```python
from build123d import *

# Parameters (mm, degrees)
SKETCH1_W           = 99
SKETCH1_H           = 126
BOSS_EXTRUDE1_DEPTH = 3
FILLET1_R           = 5
SKETCH5_R           = 18.5
SKETCH5_R_2         = 2.5
CUT_EXTRUDE4_DEPTH  = 81.176368089
SKETCH2_R           = 1.75
CUT_EXTRUDE1_DEPTH  = 81.176368089
CHAMFER1_SIZE       = 0.5
FILLET3_R           = 2
CUT_EXTRUDE3_DEPTH  = 81.176368089
SKETCH3_W           = 13.330399243
SKETCH3_H           = 8
CUT_EXTRUDE2_DEPTH  = 81.176368089
FILLET2_R           = 2.5


with BuildPart() as part:
    # Sketch1 → Boss-Extrude1 (new body)
    with BuildSketch(Plane(origin=(0, 0, 0), x_dir=(1, 0, 0), z_dir=(0, 1, 0))):
        Rectangle(SKETCH1_W, SKETCH1_H)
    extrude(amount=BOSS_EXTRUDE1_DEPTH)

    # Fillet1
    fillet1_edges = [part.edges().sort_by_distance(p)[0] for p in [
        (49.5, 1.5, 63),
        (-49.5, 1.5, 63),
        (-49.5, 1.5, -63),
        (49.5, 1.5, -63),
    ]]
    fillet(fillet1_edges, radius=FILLET1_R)

    # Sketch5 → Cut-Extrude4 (cut, through all)
    with BuildSketch(Plane(origin=(0, 3, 0), x_dir=(1, 0, 0), z_dir=(0, 1, 0))):
        with Locations(Location((0, 28, 0), (0, 0, 270))):
            Circle(SKETCH5_R)
        with Locations(Location((16, 44, 0), (0, 0, 270))):
            Circle(SKETCH5_R_2)
        with Locations(Location((16, 12, 0), (0, 0, 90))):
            Circle(SKETCH5_R_2)
        with Locations(Location((-16, 12, 0), (0, 0, 270))):
            Circle(SKETCH5_R_2)
        with Locations(Location((-16, 44, 0), (0, 0, 90))):
            Circle(SKETCH5_R_2)
    extrude(amount=-CUT_EXTRUDE4_DEPTH, mode=Mode.SUBTRACT)

    # Sketch2 → Cut-Extrude1 (cut, through all)
    with BuildSketch(Plane(origin=(0, 3, 0), x_dir=(1, 0, 0), z_dir=(0, 1, 0))):
        with Locations(Location((-43, 56.5, 0), (0, 0, 270))):
            Circle(SKETCH2_R)
        with Locations(Location((43, 56.5, 0), (0, 0, 90))):
            Circle(SKETCH2_R)
        with Locations(Location((43, -56.5, 0), (0, 0, 270))):
            Circle(SKETCH2_R)
        with Locations(Location((-43, -56.5, 0), (0, 0, 90))):
            Circle(SKETCH2_R)
    extrude(amount=-CUT_EXTRUDE1_DEPTH, mode=Mode.SUBTRACT)

    # Chamfer1
    chamfer1_edges = [part.edges().sort_by_distance(p)[0] for p in [
        (-16, 3, -41.5),
        (-16, 3, -14.5),
        (16, 3, -9.5),
        (16, 3, -46.5),
    ]]
    chamfer(chamfer1_edges, length=CHAMFER1_SIZE)

    # Fillet3
    # the kernel refuses this fillet: 2 mm, written as the material it takes off along each edge
    with BuildSketch(Plane(origin=(0, 3, -28), x_dir=(0, 0, 1), z_dir=(-1, 0, 0))) as fillet3_piece_1:
        with BuildLine():
            CenterArc((18.5 + FILLET3_R, -FILLET3_R), FILLET3_R, 90, 90)
            Line((18.5, -FILLET3_R), (18.5, 0))
            Line((18.5, 0), (18.5 + FILLET3_R, 0))
        make_face()
    revolve(axis=Axis((0, 3, -28), (0, 1, 0)), mode=Mode.SUBTRACT)

    # Sketch4 → Cut-Extrude3 (cut, through all)
    with BuildSketch(Plane(origin=(0, 3, 0), x_dir=(1, 0, 0), z_dir=(0, 1, 0))):
        with BuildLine():
            Line((-39.5, -48.833333333), (-5, -48.833333333))
            ThreePointArc((-5, -48.833333333), (-2.5, -51.333333333), (-5, -53.833333333))
            Line((-5, -53.833333333), (-39.5, -53.833333333))
            ThreePointArc((-39.5, -53.833333333), (-42, -51.333333333), (-39.5, -48.833333333))
        make_face()
        with BuildLine():
            Line((-39.5, -39.5), (-5, -39.5))
            ThreePointArc((-5, -39.5), (-2.5, -42), (-5, -44.5))
            Line((-5, -44.5), (-39.5, -44.5))
            ThreePointArc((-39.5, -44.5), (-42, -42), (-39.5, -39.5))
        make_face()
        with BuildLine():
            Line((-39.5, -30.166666667), (-5, -30.166666667))
            ThreePointArc((-5, -30.166666667), (-2.5, -32.666666667), (-5, -35.166666667))
            Line((-5, -35.166666667), (-39.5, -35.166666667))
            ThreePointArc((-39.5, -35.166666667), (-42, -32.666666667), (-39.5, -30.166666667))
        make_face()
        with BuildLine():
            Line((-39.5, -20.833333333), (-5, -20.833333333))
            ThreePointArc((-5, -20.833333333), (-2.5, -23.333333333), (-5, -25.833333333))
            Line((-5, -25.833333333), (-39.5, -25.833333333))
            ThreePointArc((-39.5, -25.833333333), (-42, -23.333333333), (-39.5, -20.833333333))
        make_face()
        with BuildLine():
            Line((-39.5, -11.5), (-5, -11.5))
            ThreePointArc((-5, -11.5), (-2.5, -14), (-5, -16.5))
            Line((-5, -16.5), (-39.5, -16.5))
            ThreePointArc((-39.5, -16.5), (-42, -14), (-39.5, -11.5))
        make_face()
        with BuildLine():
            Line((-39.5, -2.166666667), (-5, -2.166666667))
            ThreePointArc((-5, -2.166666667), (-2.5, -4.666666667), (-5, -7.166666667))
            Line((-5, -7.166666667), (-39.5, -7.166666667))
            ThreePointArc((-39.5, -7.166666667), (-42, -4.666666667), (-39.5, -2.166666667))
        make_face()
        with BuildLine():
            Line((-39.5, 7.166666667), (-14.553540997, 7.166666667))
            ThreePointArc((-14.553540997, 7.166666667), (-12.053540997, 4.666666667), (-14.553540997, 2.166666667))
            Line((-14.553540997, 2.166666667), (-39.5, 2.166666667))
            ThreePointArc((-39.5, 2.166666667), (-42, 4.666666667), (-39.5, 7.166666667))
        make_face()
        with BuildLine():
            Line((-39.5, 16.5), (-23.669600757, 16.5))
            ThreePointArc((-23.669600757, 16.5), (-21.169600757, 14), (-23.669600757, 11.5))
            Line((-23.669600757, 11.5), (-39.5, 11.5))
            ThreePointArc((-39.5, 11.5), (-42, 14), (-39.5, 16.5))
        make_face()
        with BuildLine():
            Line((-39.5, 25.833333333), (-27.101147987, 25.833333333))
            ThreePointArc((-27.101147987, 25.833333333), (-24.601147987, 23.333333333), (-27.101147987, 20.833333333))
            Line((-27.101147987, 20.833333333), (-39.5, 20.833333333))
            ThreePointArc((-39.5, 20.833333333), (-42, 23.333333333), (-39.5, 25.833333333))
        make_face()
        with BuildLine():
            Line((-39.5, 35.166666667), (-27.101147987, 35.166666667))
            ThreePointArc((-27.101147987, 35.166666667), (-24.601147987, 32.666666667), (-27.101147987, 30.166666667))
            Line((-27.101147987, 30.166666667), (-39.5, 30.166666667))
            ThreePointArc((-39.5, 30.166666667), (-42, 32.666666667), (-39.5, 35.166666667))
        make_face()
        with BuildLine():
            Line((39.5, 44.5), (23.669600757, 44.5))
            ThreePointArc((23.669600757, 44.5), (21.169600757, 42), (23.669600757, 39.5))
            Line((23.669600757, 39.5), (39.5, 39.5))
            ThreePointArc((39.5, 39.5), (42, 42), (39.5, 44.5))
        make_face()
        with BuildLine():
            Line((-39.5, 44.5), (-23.669600757, 44.5))
            ThreePointArc((-23.669600757, 44.5), (-21.169600757, 42), (-23.669600757, 39.5))
            Line((-23.669600757, 39.5), (-39.5, 39.5))
            ThreePointArc((-39.5, 39.5), (-42, 42), (-39.5, 44.5))
        make_face()
        with BuildLine():
            Line((39.5, 35.166666667), (27.101147987, 35.166666667))
            ThreePointArc((27.101147987, 35.166666667), (24.601147987, 32.666666667), (27.101147987, 30.166666667))
            Line((27.101147987, 30.166666667), (39.5, 30.166666667))
            ThreePointArc((39.5, 30.166666667), (42, 32.666666667), (39.5, 35.166666667))
        make_face()
        with BuildLine():
            Line((39.5, 25.833333333), (27.101147987, 25.833333333))
            ThreePointArc((27.101147987, 25.833333333), (24.601147987, 23.333333333), (27.101147987, 20.833333333))
            Line((27.101147987, 20.833333333), (39.5, 20.833333333))
            ThreePointArc((39.5, 20.833333333), (42, 23.333333333), (39.5, 25.833333333))
        make_face()
        with BuildLine():
            Line((39.5, 16.5), (23.669600757, 16.5))
            ThreePointArc((23.669600757, 16.5), (21.169600757, 14), (23.669600757, 11.5))
            Line((23.669600757, 11.5), (39.5, 11.5))
            ThreePointArc((39.5, 11.5), (42, 14), (39.5, 16.5))
        make_face()
        with BuildLine():
            Line((39.5, 7.166666667), (14.553540997, 7.166666667))
            ThreePointArc((14.553540997, 7.166666667), (12.053540997, 4.666666667), (14.553540997, 2.166666667))
            Line((14.553540997, 2.166666667), (39.5, 2.166666667))
            ThreePointArc((39.5, 2.166666667), (42, 4.666666667), (39.5, 7.166666667))
        make_face()
        with BuildLine():
            Line((39.5, -2.166666667), (5, -2.166666667))
            ThreePointArc((5, -2.166666667), (2.5, -4.666666667), (5, -7.166666667))
            Line((5, -7.166666667), (39.5, -7.166666667))
            ThreePointArc((39.5, -7.166666667), (42, -4.666666667), (39.5, -2.166666667))
        make_face()
        with BuildLine():
            Line((39.5, -11.5), (5, -11.5))
            ThreePointArc((5, -11.5), (2.5, -14), (5, -16.5))
            Line((5, -16.5), (39.5, -16.5))
            ThreePointArc((39.5, -16.5), (42, -14), (39.5, -11.5))
        make_face()
        with BuildLine():
            Line((39.5, -20.833333333), (5, -20.833333333))
            ThreePointArc((5, -20.833333333), (2.5, -23.333333333), (5, -25.833333333))
            Line((5, -25.833333333), (39.5, -25.833333333))
            ThreePointArc((39.5, -25.833333333), (42, -23.333333333), (39.5, -20.833333333))
        make_face()
        with BuildLine():
            Line((39.5, -30.166666667), (5, -30.166666667))
            ThreePointArc((5, -30.166666667), (2.5, -32.666666667), (5, -35.166666667))
            Line((5, -35.166666667), (39.5, -35.166666667))
            ThreePointArc((39.5, -35.166666667), (42, -32.666666667), (39.5, -30.166666667))
        make_face()
        with BuildLine():
            Line((39.5, -39.5), (5, -39.5))
            ThreePointArc((5, -39.5), (2.5, -42), (5, -44.5))
            Line((5, -44.5), (39.5, -44.5))
            ThreePointArc((39.5, -44.5), (42, -42), (39.5, -39.5))
        make_face()
        with BuildLine():
            Line((39.5, -48.833333333), (5, -48.833333333))
            ThreePointArc((5, -48.833333333), (2.5, -51.333333333), (5, -53.833333333))
            Line((5, -53.833333333), (39.5, -53.833333333))
            ThreePointArc((39.5, -53.833333333), (42, -51.333333333), (39.5, -48.833333333))
        make_face()
        with BuildLine():
            Line((14.553540997, 53.833333333), (39.5, 53.833333333))
            ThreePointArc((39.5, 53.833333333), (42, 51.333333333), (39.5, 48.833333333))
            Line((39.5, 48.833333333), (14.553540997, 48.833333333))
            ThreePointArc((14.553540997, 48.833333333), (12.053540997, 51.333333333), (14.553540997, 53.833333333))
        make_face()
    extrude(amount=-CUT_EXTRUDE3_DEPTH, mode=Mode.SUBTRACT)

    # Sketch3 → Cut-Extrude2 (cut, through all)
    with BuildSketch(Plane(origin=(0, 3, 0), x_dir=(1, 0, 0), z_dir=(0, 1, 0))):
        with Locations((-27.834800378, 59)):
            Rectangle(SKETCH3_W, SKETCH3_H)
    extrude(amount=-CUT_EXTRUDE2_DEPTH, mode=Mode.SUBTRACT)

    # Fillet2
    fillet2_edges = [part.edges().sort_by_distance(p)[0] for p in [
        (-34.5, 1.5, -55),
        (-34.5, 1.5, -63),
        (-21.169600757, 1.5, -63),
        (-21.169600757, 1.5, -55),
    ]]
    fillet(fillet2_edges, radius=FILLET2_R)


solid = part.part
```
Geometry: final body of the model. Coordinates: model frame, mm. Round coordinates to 2 decimals unless told otherwise and drop trailing zeros. Order: outer loops, then holes, each group sorted by start corner. A loop starts at its lowest first (then second) coordinate and runs counter-clockwise, first axis right, second up. Notation, with made-up numbers: (42, 52.5) -> (47, 52.5) arc R12 cw to (47, 58.5) -> close; hole circle Ø11 at (16, -16.75). An arc over 180 degrees is marked (long way). Use CSV: the item, a comma, the result in double quotes. Start each with the question number.
1) Section D-D (y = 1.5). State how many separate pieces and enclosed holes the cut face has, and give its area (3 significant figures).
2) Draft query along Z for faces 1 (the face through (-31, 2, -39.5)), 2 (the face through (48, 1.52, 61.57)), 3 (the face through (-1, 3, -1)). Return one class per face: +Z half, -Z half, draft (parallel to the pull), parting line (faces both ways), or undercut.
3) Material intervals for line 1 along X through (y, z) = (0.85, 5); line 2 along X through (y, z) = (0.6, -27.5); line 3 along X through (y, z) = (2, -12), sorted ascending. Write a range as from..to.
4) First-contact query: pin 1 Ø4.5 at (x, z) = (16, -12) entering from -Y. Flat tip, straight axial feed; report the tip coordinate or a pass-through.
5) Section A-A (z = 56.5). Return the cut outline in (x, y).
6) Section B-B (z = -28). Return the cut outline in (x, y), and give its area (3 significant figures).
7) Section C-C (z = 23). Return the cut outline in (x, y), and give its area (3 significant figures).
Returned:
1,separate pieces,"1"
1,enclosed holes,"32"
1,area,"7,690 mm²"
2,face 1,"undercut"
2,face 2,"+Z half"
2,face 3,"draft"
3,line 1,"x = -49.5..-41.98, -2.52..2.52, 41.98..49.5"
3,line 2,"x = -49.5..-18.49, 18.49..49.5"
3,line 3,"x = -49.5..-41, -22.17..-18.5, -13.5..-9.81, 9.81..13.5, 18.5..22.17, 41..49.5"
4,pin 1,"passes through"
5,outline,"(-49.5, 0) -> (-44.75, 0) -> (-44.75, 3) -> (-49.5, 3) -> close; (-41.25, 0) -> (41.25, 0) -> (41.25, 3) -> (-41.25, 3) -> close; (44.75, 0) -> (49.5, 0) -> (49.5, 3) -> (44.75, 3) -> close"
6,outline,"(-49.5, 0) -> (-18.5, 0) -> (-18.5, 1) arc R2 ccw to (-20.5, 3) -> (-49.5, 3) -> close; (18.5, 0) -> (49.5, 0) -> (49.5, 3) -> (20.5, 3) arc R2 ccw to (18.5, 1) -> close"
6,area,"184 mm²"
7,outline,"(-49.5, 0) -> (-41.98, 0) -> (-41.98, 3) -> (-49.5, 3) -> close; (-2.52, 0) -> (2.52, 0) -> (2.52, 3) -> (-2.52, 3) -> close; (41.98, 0) -> (49.5, 0) -> (49.5, 3) -> (41.98, 3) -> close"
7,area,"60.3 mm²"
